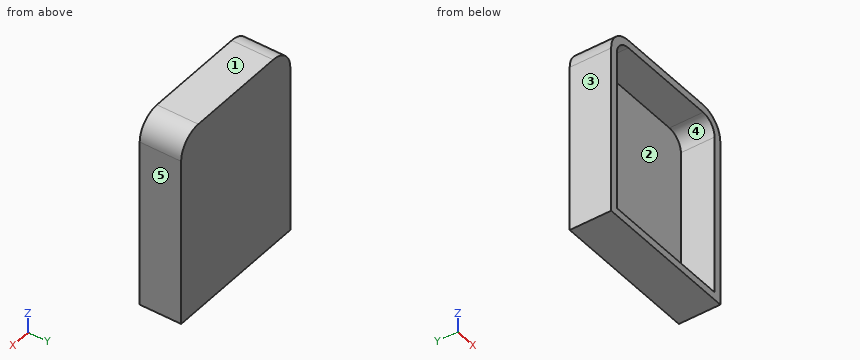
from build123d import *

# Parameters (mm, degrees)
F1_DEPTH = 8
F2_DEPTH = 1.5


# Not quite as in the source:
# - a feature names something its author has since deleted; it is built from what else it names


with BuildPart() as f1:
    # F0 (on Front) → F1 (new body)
    with BuildSketch(Plane.XZ):
        with BuildLine():
            Line((-27.1, 31.2), (-27.1, -1.5))
            Line((-27.1, -1.5), (1.5, -1.5))
            Line((1.5, -1.5), (1.5, 31.2))
            ThreePointArc((1.5, 31.2), (0.1819805153, 34.3819805153), (-3, 35.7))
            Line((-3, 35.7), (-22.6, 35.7))
            ThreePointArc((-22.6, 35.7), (-25.7819805153, 34.3819805153), (-27.1, 31.2))
        make_face()
        with BuildLine():
            ThreePointArc((-25.6, 31.2), (-24.7213203436, 33.3213203436), (-22.6, 34.2))
            Line((-22.6, 34.2), (-3, 34.2))
            ThreePointArc((-3, 34.2), (-0.8786796564, 33.3213203436), (0, 31.2))
            Line((0, 31.2), (0, 0))
            Line((0, 0), (-25.6, 0))
            Line((-25.6, 0), (-25.6, 31.2))
        make_face(mode=Mode.SUBTRACT)
    extrude(amount=F1_DEPTH)

    # F0 (on Front) → F2 (join)
    with BuildSketch(Plane.XZ):
        with BuildLine():
            Line((-3, 34.2), (-22.6, 34.2))
            ThreePointArc((-22.6, 34.2), (-24.7213203436, 33.3213203436), (-25.6, 31.2))
            Line((-25.6, 31.2), (-25.6, 0))
            Line((-25.6, 0), (0, 0))
            Line((0, 0), (0, 31.2))
            ThreePointArc((0, 31.2), (-0.8786796564, 33.3213203436), (-3, 34.2))
        make_face()
    extrude(amount=F2_DEPTH)


solid = f1.part
Source: CAD feature listing. Evaluate the final solid. Frame: model axes, mm. Face numbers are marked on the shaded views. A direction names the side the tool comes from. Round coordinates to 2 decimals unless told otherwise and drop trailing zeros. Loops run counter-clockwise (first coordinate to the right, second up) from the corner with the lowest first, then second, coordinate; pieces in that order, holes last. Notation, with made-up numbers: (25, -8) - (58, -8) arc R10 ccw to (58, 0) - close; hole circle Ø11 at (-6.75, 79.25). An arc over 180 degrees is marked (long way). Write item = value, one per line. Start each with the question number.
(1) Section query B-B, the plane y = -4.5. Output: boundary loops of the cut face in (x, z).
(2) Set-up query: the marked faces 4 and 5. Return all of +Z, -Z, +X, -X, +Y, -Y with unobstructed straight access to the full face (end or side cutting, diameter ignored); none if empty.
(3) Section query C-C, the plane x = -12.5. Output: boundary loops of the cut face in (y, z), plus the area to 3 significant figures.
(4) Section query A-A, the plane z = 16. Output: boundary loops of the cut face in (x, y).
(5) Pin query (flat end, axial travel): pin 1 (2 mm diameter, centred on x = -21.5, z = 15.5, fed in from -Y). Return the tip coordinate at first contact, or that it passes through.
(6) Ray query, line 1 along Z through (x, y) = (-4.25, -4); line 2 along X through (y, z) = (-7, 4); line 3 along Y through (x, z) = (-11, 1.5). Return the intervals inside material, ascending. Write a range as from..to.
(7) Pull-direction query (Z, two-part tool) for the marked faces 1, 2 and 3; classes: +Z half, -Z half, draft (parallel to the pull), parting line (faces both ways), or undercut.
Conclusion:
q1.outline = (-27.1, -1.5) - (1.5, -1.5) - (1.5, 31.2) arc R4.5 ccw to (-3, 35.7) - (-22.6, 35.7) arc R4.5 ccw to (-27.1, 31.2) - close; hole (-25.6, 0) - (0, 0) - (0, 31.2) arc R3 ccw to (-3, 34.2) - (-22.6, 34.2) arc R3 ccw to (-25.6, 31.2) - close
q2.face_4 = -Y
q2.face_5 = +Z, -Z, +X, +Y, -Y
q3.outline = (-8, -1.5) - (0, -1.5) - (0, 35.7) - (-8, 35.7) - (-8, 34.2) - (-1.5, 34.2) - (-1.5, 0) - (-8, 0) - close
q3.area = 75.3 mm2
q4.outline = (-27.1, -8) - (-25.6, -8) - (-25.6, -1.5) - (0, -1.5) - (0, -8) - (1.5, -8) - (1.5, 0) - (-27.1, 0) - close
q5.pin_1 = -1.5
q6.line_1 = -1.5..0, 34.2..35.7
q6.line_2 = -27.1..-25.6, 0..1.5
q6.line_3 = -1.5..0
q7.face_1 = +Z half
q7.face_2 = undercut
q7.face_3 = draft
